Can you work these out from the drawing? Everything is in mm from the part's minimum corner. Coordinates: 2 decimals unless noted, no trailing zeros. Loops run counter-clockwise (first coordinate to the right, second up) from the corner with the lowest first, then second, coordinate; pieces in that order, holes last. Notation, with made-up numbers: (66.25, -19.5) -> (116.25, -19.5) arc R13 cw to (116.25, -10.5) -> close; hole circle Ø9 at (30.5, 78.25). An arc over 180 degrees is marked (long way). Use one line per item in the form item = value. Start each with the question number.
(1) Imagine slicing it at A-A (x = 24.5). List the corners of the cut face in (y, z) for me.
(2) Imagine slicing it at D-D (x = 3.5). List the corners of the cut face in (y, z) for me, plus the area to 3 significant figures.
(3) I need wall thicknesses on line 1 (X direction, y = 2.25, z = 22.5); line 2 (X direction, y = 5.5, z = 86); line 3 (X direction, y = 5.25, z = 28.5). Which ranges of each line are inside material? Lowest first, please. Write a range as [from, to].
(4) Imagine slicing it at C-C (y = 5.5). List the corners of the cut face in (x, z) for me.
(5) Imagine slicing it at B-B (z = 117.5). List the corners of the cut face in (x, y) for me.
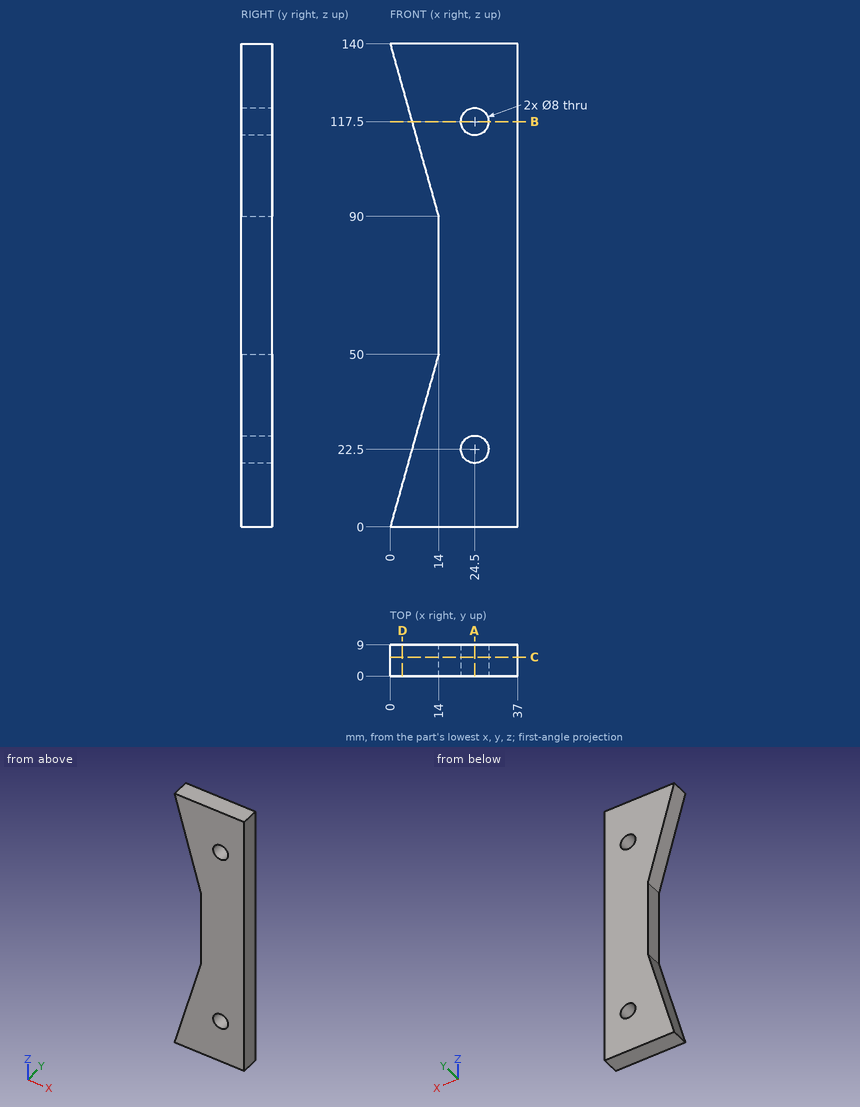
Worked out:
q1.outline = (0, 0) -> (9, 0) -> (9, 18.5) -> (0, 18.5) -> close; (0, 26.5) -> (9, 26.5) -> (9, 113.5) -> (0, 113.5) -> close; (0, 121.5) -> (9, 121.5) -> (9, 140) -> (0, 140) -> close
q2.outline = (0, 0) -> (9, 0) -> (9, 12.5) -> (0, 12.5) -> close; (0, 127.5) -> (9, 127.5) -> (9, 140) -> (0, 140) -> close
q2.area = 225 mm2
q3.line_1 = [6.3, 20.5], [28.5, 37]
q3.line_2 = [14, 37]
q3.line_3 = [7.98, 37]
q4.outline = (0, 0) -> (37, 0) -> (37, 140) -> (0, 140) -> (14, 90) -> (14, 50) -> close; hole circle Ø8 at (24.5, 22.5); hole circle Ø8 at (24.5, 117.5)
q5.outline = (6.3, 0) -> (20.5, 0) -> (20.5, 9) -> (6.3, 9) -> close; (28.5, 0) -> (37, 0) -> (37, 9) -> (28.5, 9) -> close
